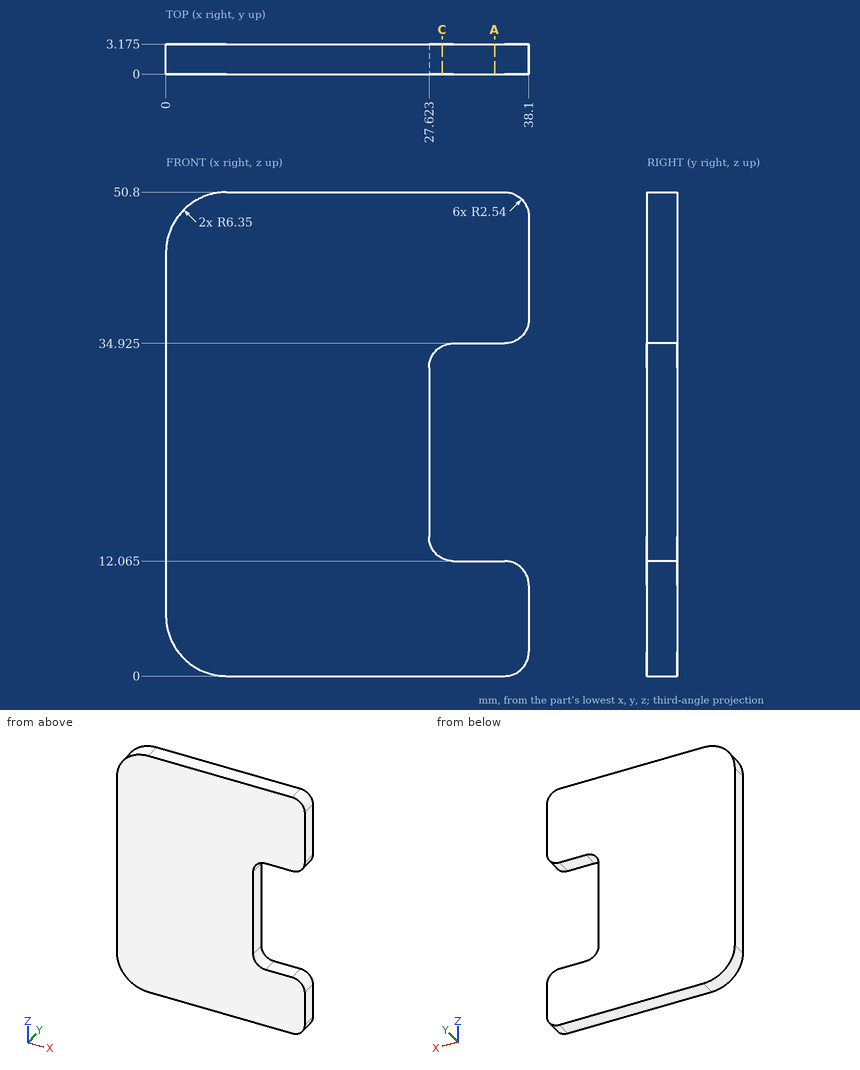
Study the drawing (mm; zero at the part's minimum x, y, z) and answer. Round coordinates to 2 decimals unless told otherwise and drop trailing zeros. Write each loop counter-clockwise with the first axis right and the second up, starting at its lowest first coordinate (ties: lowest second). Pieces come first, ordered by that corner, then holes. Notation, with made-up numbers: (14, 16.25) -> (25, 16.25) arc R26 cw to (25, 54.25) -> close; hole circle Ø10 at (7, 11.25). An arc over 180 degrees is marked (long way). Answer as CSV lines item,"result". Start each with the question number.
(1) Find the intervals of material crossed by probe 1 along Z at (x, y) = (32, 2.45) (1 decimal); probe 2 along Z at (x, y) = (6, 2.55); probe 3 along X at (y, z) = (0.35, 30.5), in increasing order.
(2) This flat-tipped pin is pushed along its axis until it touches: pin 1 (6 mm diameter, centred on x = 9, z = 17, fed in from -Y). Where does it stop, or does it pass through?
(3) The part is cut by section C-C, the plane x = 29. Give the vertices of the cut face in (y, z) (1 decimal).
(4) The part is cut by section A-A, the plane x = 34.5. Give the vertices of the cut face in (y, z) (1 decimal).
Output values:
1,probe 1,"z = 0 to 12.1, 34.9 to 50.8"
1,probe 2,"z = 0.01 to 50.79"
1,probe 3,"x = 0 to 27.62"
2,pin 1,"stops at y = 0"
3,outline,"(0, 0) -> (3.2, 0) -> (3.2, 12.3) -> (0, 12.3) -> close; (0, 34.6) -> (3.2, 34.6) -> (3.2, 50.8) -> (0, 50.8) -> close"
4,outline,"(0, 0) -> (3.2, 0) -> (3.2, 12.1) -> (0, 12.1) -> close; (0, 34.9) -> (3.2, 34.9) -> (3.2, 50.8) -> (0, 50.8) -> close"
